Could you check a few things on this model? Use its own coordinates, in mm. A direction names the side the tool comes from. Give positions to 0.01 mm unless a question says otherwise; leave off trailing zeros. Order: outer loops, then holes, each group sorted by start corner. A loop starts at its lowest first (then second) coordinate and runs counter-clockwise, first axis right, second up. Notation, with made-up numbers: (-25, 55) -> (25, 55) arc R21 cw to (25, 64) -> close; hole circle Ø6 at (0.25, -22.5). An arc over 180 degrees is marked (long way). One line per item, written item: value.
```python
from build123d import *

# Parameters (mm, degrees)
F0_R     = 12.5
F1_DEPTH = 105
F3_DEPTH = 52
F4_R     = 3
F6_D     = 4
F6_DEPTH = 20
F6_TIP   = 1.2017212381
F7_D     = 4
F7_DEPTH = 20
F7_START = 11
F7_TIP   = 1.2017212381
F8_R     = 1


with BuildPart() as f1:
    # F0 (on Top) → F1 (new body)
    with BuildSketch(Plane.XY):
        Circle(F0_R)
    extrude(amount=F1_DEPTH)

    # F2 (on face) → F3 (join)
    with BuildSketch(Plane.XY.offset(105)):
        with BuildLine():
            Line((11.2334422785, -5.4826795069), (-11.2334422785, -5.4826795069))
            ThreePointArc((-11.2334422785, -5.4826795069), (0, -12.5), (11.2334422785, -5.4826795069))
        make_face()
        with BuildLine():
            ThreePointArc((11.2164688996, 5.5173204931), (0, 12.5), (-11.2164688996, 5.5173204931))
            Line((-11.2164688996, 5.5173204931), (11.2164688996, 5.5173204931))
        make_face()
    extrude(amount=F3_DEPTH)

    # F4
    f4_edges = [f1.edges().sort_by_distance(p)[0] for p in [
        (-12.5, 0, 0),
    ]]
    fillet(f4_edges, radius=F4_R)

    # F6 (one way)
    with BuildSketch(Plane.XZ.offset(-5.5173204931)):
        with Locations((0, 147)):
            Circle(F6_D / 2)
    extrude(amount=-F6_DEPTH, mode=Mode.SUBTRACT)
    with Locations(Plane.XZ.offset(-5.5173204931)):
        with Locations((0, 147)):
            with Locations((0, 0, -(F6_DEPTH + F6_TIP / 2))):  # 118° drill point
                Cone(0, F6_D / 2, F6_TIP, mode=Mode.SUBTRACT)

    # F7
    # its depths count from where the whole tool has entered the part; down to there all is cleared
    with Locations(Plane(origin=(0, 5.5173204931, 0), x_dir=(1, 0, 0), z_dir=(0, 1, 0)).offset(-F7_START)):
        with Locations((0, -147)):
            Hole(F7_D / 2, depth=F7_DEPTH)
            with Locations((0, 0, -(F7_DEPTH + F7_TIP / 2))):  # 118° drill point
                Cone(0, F7_D / 2, F7_TIP, mode=Mode.SUBTRACT)

    # F8
    f8_edges = [f1.edges().sort_by_distance(p)[0] for p in [
        (0, 12.5, 157),
        (0, -12.5, 157),
    ]]
    fillet(f8_edges, radius=F8_R)


solid = f1.part
```
1) Suppose I cut it at B-B, the plane z = 107. Write out the boundary of the cut face in (x, y).
Answer below:
outline: (-11.23, -5.48) arc R12.5 ccw to (11.23, -5.48) -> close; (-11.22, 5.52) -> (11.22, 5.52) arc R12.5 ccw to start
2) Suppose I cut it at D-D, the plane z = 147. Write out the boundary of the cut face in (x, y).
Answer below:
outline: (-11.23, -5.48) arc R12.5 ccw to (-2, -12.34) -> (-2, -5.48) -> close; (-11.22, 5.52) -> (-2, 5.52) -> (-2, 12.34) arc R12.5 ccw to start; (2, -12.34) arc R12.5 ccw to (11.23, -5.48) -> (2, -5.48) -> close; (2, 5.52) -> (11.22, 5.52) arc R12.5 ccw to (2, 12.34) -> close
3) For P1, Ø10, axis at x = -9.5, z = 95, coming from the -Y side; P2, Ø10, axis at x = -7, z = 19, coming from the -Y side; P3, Ø4, axis at y = -2.5, z = 43.5, coming from the +X side, each with a flat end and sliding along its axis, tell me the tip position at first contact or that it passes through.
Answer below:
P1: stops at y = -11.66
P2: stops at y = -12.34
P3: stops at x = 12.49
4) For faces 1 (the flat face through (0, -8, 157)), 2 (the flat face through (0, 5.517, 131)), which set-ups out of +Z, -Z, +X, -X, +Y, -Y let a thin tool reach every point of the face, with its end or its side?
Answer below:
face 1: +Z, +X, -X, +Y, -Y
face 2: +Z, +X, -X
5) We'd pull the mould along Z, two halves only. Please class faces 3 (the cylindrical face through (-0.923, -9.043, 148.774)), 4 (the flat face through (0, 0, 0)), 5 (the flat face through (0, 0, 105)), 6 (the flat face through (0, -5.483, 131)): +Z half, -Z half, draft (parallel to the pull), parting line (faces both ways), or undercut.
Answer below:
face 3: undercut
face 4: -Z half
face 5: +Z half
face 6: draft
6) Suppose I cut it at C-C, the plane y = 0. Write out the boundary of the cut face in (x, z).
Answer below:
outline: (-12.5, 3) arc R3 ccw to (-9.5, 0) -> (9.5, 0) arc R3 ccw to (12.5, 3) -> (12.5, 105) -> (-12.5, 105) -> close
7) If I drill on line 1 along Z through (x, y) = (0, -8.25); line 2 along X through (y, z) = (7, 147); line 3 along X through (y, z) = (-8.25, 147), over which ranges is the centre line in solid material (lowest first)?
Answer below:
line 1: z = 0 to 145, 149 to 157
line 2: x = -10.36 to -2, 2 to 10.36
line 3: x = -9.39 to -2, 2 to 9.39
8) Suppose I cut it at A-A, the plane x = 0. Write out the boundary of the cut face in (y, z).
Answer below:
outline: (-12.5, 3) arc R3 ccw to (-9.5, 0) -> (9.5, 0) arc R3 ccw to (12.5, 3) -> (12.5, 145) -> (5.52, 145) -> (5.52, 105) -> (-5.48, 105) -> (-5.48, 145) -> (-12.5, 145) -> close; (-12.5, 149) -> (-5.48, 149) -> (-5.48, 157) -> (-11.5, 157) arc R1 ccw to (-12.5, 156) -> close; (5.52, 149) -> (12.5, 149) -> (12.5, 156) arc R1 ccw to (11.5, 157) -> (5.52, 157) -> close
